For this review, take the finished solid that the model builds, in its own axes (mm). Round coordinates to 2 decimals unless told otherwise and drop trailing zeros. Loops run counter-clockwise (first coordinate to the right, second up) from the corner with the lowest first, then second, coordinate; pieces in that order, holes last.
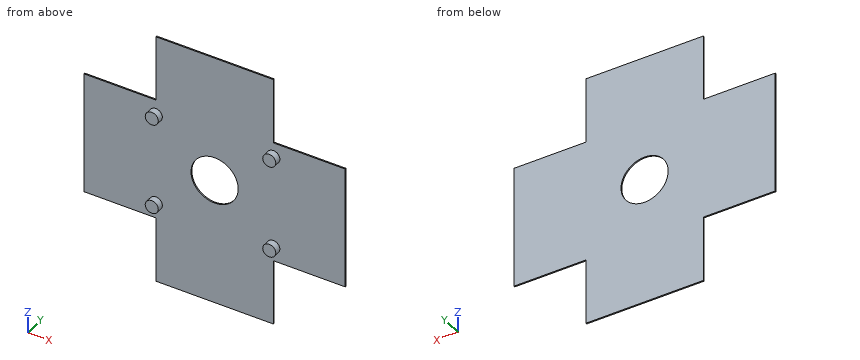
```python
from build123d import *

# Parameters (mm, degrees)
BOSS_EXTRUDE1_DEPTH = 2
SKETCH2_R           = 36.15
CUT_EXTRUDE1_DEPTH  = 542.526676351
SKETCH3_R           = 10
BOSS_EXTRUDE2_DEPTH = 10


with BuildPart() as part:
    # Sketch1 → Boss-Extrude1 (new body)
    with BuildSketch(Plane.XZ.offset(167)):
        Polygon((279.299936853, -275.420908514), (389.299936853, -275.420908514), (389.299936853, -87.420908514), (279.299936853, -87.420908514), (279.299936853, 13.579091486), (99.299936853, 13.579091486), (99.299936853, -87.420908514), (-10.700063147, -87.420908514), (-10.700063147, -275.420908514), (99.299936853, -275.420908514), (99.299936853, -376.420908514), (279.299936853, -376.420908514), align=None)
    extrude(amount=-BOSS_EXTRUDE1_DEPTH)

    # Sketch2 → Cut-Extrude1 (cut, through all)
    with BuildSketch(Plane(origin=(0, -165, 0), x_dir=(1, 0, 0), z_dir=(0, 1, 0))):
        with Locations(Location((189.299936853, 181.420908514, 0), (0, 0, 270))):
            Circle(SKETCH2_R)
    extrude(amount=-CUT_EXTRUDE1_DEPTH, mode=Mode.SUBTRACT)

    # Sketch3 → Boss-Extrude2 (add)
    with BuildSketch(Plane.XZ.offset(167)):
        with Locations(Location((99.299936853, -110.952514015, 0), (0, 0, 90))):
            Circle(SKETCH3_R)
        with Locations(Location((279.299936853, -109.641474118, 0), (0, 0, 90))):
            Circle(SKETCH3_R)
        with Locations(Location((279.299936853, -253.20034291, 0), (0, 0, 90))):
            Circle(SKETCH3_R)
        with Locations(Location((99.299936853, -251.889303012, 0), (0, 0, 90))):
            Circle(SKETCH3_R)
    extrude(amount=BOSS_EXTRUDE2_DEPTH)


solid = part.part
```
(1) Insertion check: pin 1 Ø1 at (x, y) = (23.5, -166.5) entering from +Z; pin 2 Ø1.5 at (y, z) = (-171.5, -248) entering from -X; pin 3 Ø0.6 at (y, z) = (-165.5, -26.5) entering from +X. Each pin has a flat end and moves straight along its axis. Give the tip position at first contact, or say it passes through.
(2) Add section A-A (y = -172.5). Give the boundary of the cut face in (x, z), plus the area to 3 significant figures.
(3) Add section C-C (z = -172). Give the boundary of the cut face in (x, y).
(4) For L1, parallel to Y at x = 362, z = -111.5; L2, parallel to Z at x = 291, y = -166.75; L3, parallel to X at y = -167.75, z = -117.5, list the stretches that pass through material, from the lowest coordinate up.
(5) Add section D-D (z = -128.5). Give the boundary of the cut face in (x, y).
(6) Add section B-B (x = 216). Give the boundary of the cut face in (y, z).
Outcome:
1. pin 1: stops at z = -87.42
1. pin 2: stops at x = 89.81
1. pin 3: stops at x = 279.3
2. outline: circle Ø20 at (99.3, -251.89); circle Ø20 at (99.3, -110.95); circle Ø20 at (279.3, -253.2); circle Ø20 at (279.3, -109.64)
2. area: 1,260 mm2
3. outline: (-10.7, -167) - (154.4, -167) - (154.4, -165) - (-10.7, -165) - close; (224.2, -167) - (389.3, -167) - (389.3, -165) - (224.2, -165) - close
4. L1: y = -167 to -165
4. L2: z = -275.42 to -87.42
4. L3: x = 91.74 to 106.86, 273.12 to 285.48
5. outline: (-10.7, -167) - (389.3, -167) - (389.3, -165) - (-10.7, -165) - close
6. outline: (-167, -376.42) - (-165, -376.42) - (-165, -205.79) - (-167, -205.79) - close; (-167, -157.05) - (-165, -157.05) - (-165, 13.58) - (-167, 13.58) - close
